from build123d import *

# Parameters (mm, degrees)
F1_DEPTH = 480
F2_R     = 9
F3_DEPTH = 10
F4_R     = 15
F5_DEPTH = 10
F6_R     = 10
F7_R     = 20


with BuildPart() as f1:
    # F0 (on Front) → F1 (new body, symmetric)
    with BuildSketch(Plane.XZ):
        Polygon((0, 200), (0, 0), (120, 0), (120, 10), (10, 10), (10, 200), align=None)
    extrude(amount=F1_DEPTH, both=True)

    # F2 (on face) → F3 (cut, through all)
    with BuildSketch(Plane.YZ.offset(10)):
        with Locations((-373, 170)):
            Circle(F2_R)
        with BuildLine():
            ThreePointArc((-434, 179), (-436.6360389693, 185.3639610307), (-443, 188))
            ThreePointArc((-443, 188), (-449.3639610307, 185.3639610307), (-452, 179))
            Line((-452, 179), (-452, 161))
            ThreePointArc((-452, 161), (-449.3639610307, 154.6360389693), (-443, 152))
            ThreePointArc((-443, 152), (-436.6360389693, 154.6360389693), (-434, 161))
            Line((-434, 161), (-434, 179))
        make_face()
        with BuildLine():
            ThreePointArc((443, 188), (436.6360389693, 185.3639610307), (434, 179))
            Line((434, 179), (434, 161))
            ThreePointArc((434, 161), (436.6360389693, 154.6360389693), (443, 152))
            ThreePointArc((443, 152), (449.3639610307, 154.6360389693), (452, 161))
            Line((452, 161), (452, 179))
            ThreePointArc((452, 179), (449.3639610307, 185.3639610307), (443, 188))
        make_face()
    extrude(amount=-F3_DEPTH, mode=Mode.SUBTRACT)

    # F4 (on face) → F5 (cut, through all)
    with BuildSketch(Plane.XY.offset(10)):
        with Locations((80, -250)):
            Circle(F4_R)
        with Locations((80, 250)):
            Circle(F4_R)
    extrude(amount=-F5_DEPTH, mode=Mode.SUBTRACT)

    # F6
    f6_edges = [f1.edges().sort_by_distance(p)[0] for p in [
        (10, 0, 10),
    ]]
    fillet(f6_edges, radius=F6_R)

    # F7
    f7_edges = [f1.edges().sort_by_distance(p)[0] for p in [
        (0, 0, 0),
    ]]
    fillet(f7_edges, radius=F7_R)


solid = f1.part
The model under review builds one solid part; all positions refer to its coordinate system, in mm. A direction names the side the tool comes from. Give positions to 0.01 mm unless a question says otherwise; leave off trailing zeros. Loops run counter-clockwise (first coordinate to the right, second up) from the corner with the lowest first, then second, coordinate; pieces in that order, holes last. Notation, with made-up numbers: (84.5, 70.25) -> (95.5, 70.25) arc R8 ccw to (95.5, 84.25) -> close; hole circle Ø11 at (39.5, -31). An arc over 180 degrees is marked (long way). Write each question's results on one line, items separated by ' | '.
1) Insertion check: pin 1 Ø12 at (y, z) = (162, 62) entering from +X; pin 2 Ø18 at (x, y) = (80, 250) entering from -Z; pin 3 Ø20.5 at (y, z) = (-373, 170) entering from -X; pin 4 Ø4 at (x, y) = (63, 261.5) entering from +Z. Each pin has a flat end and moves straight along its axis. Give the tip position at first contact, or say it passes through.
Conclusion:
pin 1: stops at x = 10 | pin 2: passes through | pin 3: stops at x = 0 | pin 4: stops at z = 10
2) For line 1 along Y through (x, z) = (80, 5); line 2 along X through (y, z) = (414, 108.5), list the stretches that pass through material, from the lowest coordinate up. Write a range as from..to.
Conclusion:
line 1: y = -480..-265, -235..235, 265..480 | line 2: x = 0..10
3) Tool access review of faces 4 (the face through (69, -7, 0)), 5 (the face through (71, -7, 10)): name each direction out of +Z, -Z, +X, -X, +Y, -Y from which nothing blocks a thin tool from reaching the whole face with its end or side.
Conclusion:
face 4: -Z, +X, -X, +Y, -Y | face 5: +Z, +X, +Y, -Y
4) Take a section at D-D, the plane y = -142.5. Give the boundary of the cut face in (x, z), plus the area to 3 significant figures.
Conclusion:
outline: (0, 20) arc R20 ccw to (20, 0) -> (120, 0) -> (120, 10) -> (20, 10) arc R10 cw to (10, 20) -> (10, 200) -> (0, 200) -> close | area: 3,040 mm^2
5) Draft analysis for pull direction Y (two halves, no side actions). For faces 1 (the face through (76.748, -264.643, 5.07)), 2 (the face through (10, -7, 109)), 3 (the face through (6, 480, 71)), state which applies: pulls with the +Y half, pulls with the -Y half, needs draft (parallel to the pull), parting line crosses it, or undercut.
Conclusion:
face 1: undercut | face 2: needs draft | face 3: pulls with the +Y half
6) Take a section at A-A, the plane y = 250. Give the boundary of the cut face in (x, z).
Conclusion:
outline: (0, 20) arc R20 ccw to (20, 0) -> (65, 0) -> (65, 10) -> (20, 10) arc R10 cw to (10, 20) -> (10, 200) -> (0, 200) -> close; (95, 0) -> (120, 0) -> (120, 10) -> (95, 10) -> close
7) Take a section at C-C, the plane x = 80. Give the boundary of the cut face in (y, z), plus the area to 3 significant figures.
Conclusion:
outline: (-480, 0) -> (-265, 0) -> (-265, 10) -> (-480, 10) -> close; (-235, 0) -> (235, 0) -> (235, 10) -> (-235, 10) -> close; (265, 0) -> (480, 0) -> (480, 10) -> (265, 10) -> close | area: 9,000 mm^2
8) Take a section at B-B, the plane z = 170. Give the boundary of the cut face in (x, y), plus the area to 3 significant figures.
Conclusion:
outline: (0, -480) -> (10, -480) -> (10, -452) -> (0, -452) -> close; (0, -434) -> (10, -434) -> (10, -382) -> (0, -382) -> close; (0, -364) -> (10, -364) -> (10, 434) -> (0, 434) -> close; (0, 452) -> (10, 452) -> (10, 480) -> (0, 480) -> close | area: 9,060 mm^2
